Can you work these out from the model? Positions are in its coordinate system, mm. Face numbers are marked on the shaded views. Give positions to 0.01 mm unless a question says otherwise; leave off trailing zeros. Write each loop counter-clockwise with the first axis right and the second up, starting at its lowest first coordinate (ties: lowest second). Pieces come first, ordered by that corner, then holes. Notation, with made-up numbers: (87, -14) -> (122, -14) arc R14 ccw to (122, -4) -> close; hole circle Ø11 at (15.5, -39.75). An arc over 180 degrees is marked (long way). One line per item, written item: value.
from build123d import *

# Parameters (mm, degrees)
BASE_PLATE_R    = 1.6
EXTRUDE_1_DEPTH = 1.55
FILLET_1_R      = 1
SKETCH_1_R      = 3.25
SKETCH_1_R_2    = 3.5
EXTRUDE_2_DEPTH = 4.5
SKETCH_1_3_R    = 2.4
EXTRUDE_3_DEPTH = 2
SKETCH_1_4_R    = 2.5
EXTRUDE_4_DEPTH = 1.2


with BuildPart() as part:
    # Base plate → Extrude 1 (new body)
    with BuildSketch(Plane(origin=(0, 0, 0), x_dir=(1, 0, 0), z_dir=(0, 1, 0))):
        with BuildLine():
            ThreePointArc((-38.1, -33.9), (-36.869848481, -36.869848481), (-33.9, -38.1))
            Line((-33.9, -38.1), (33.9, -38.1))
            ThreePointArc((33.9, -38.1), (36.869848481, -36.869848481), (38.1, -33.9))
            Line((38.1, -33.9), (38.1, 33.9))
            ThreePointArc((38.1, 33.9), (36.869848481, 36.869848481), (33.9, 38.1))
            Line((33.9, 38.1), (-0.9, 38.1))
            Line((-0.9, 38.1), (-0.9, 27.4))
            ThreePointArc((-0.9, 27.4), (-2.9, 25.4), (-4.9, 27.4))
            Line((-4.9, 27.4), (-4.9, 38.1))
            Line((-4.9, 38.1), (-33.9, 38.1))
            ThreePointArc((-33.9, 38.1), (-36.869848481, 36.869848481), (-38.1, 33.9))
            Line((-38.1, 33.9), (-38.1, -33.9))
        make_face()
        with Locations(Location((-33.9, -33.9, 0), (0, 0, 90))):
            Circle(BASE_PLATE_R, mode=Mode.SUBTRACT)
        with Locations(Location((33.9, -33.9, 0), (0, 0, 90))):
            Circle(BASE_PLATE_R, mode=Mode.SUBTRACT)
        with Locations(Location((-33.9, 33.9, 0), (0, 0, 90))):
            Circle(BASE_PLATE_R, mode=Mode.SUBTRACT)
        with Locations(Location((33.9, 33.9, 0), (0, 0, 90))):
            Circle(BASE_PLATE_R, mode=Mode.SUBTRACT)
    extrude(amount=EXTRUDE_1_DEPTH)

    # Fillet 1
    fillet_1_edges = [part.edges().sort_by_distance(p)[0] for p in [
        (-0.9, 0.775, -38.1),
        (-4.9, 0.775, -38.1),
    ]]
    fillet(fillet_1_edges, radius=FILLET_1_R)

    # Sketch 1 → Extrude 2 (add)
    with BuildSketch(Plane.XZ):
        with Locations(Location((-22.7, -3.07, 0), (0, 0, 90))):
            Circle(SKETCH_1_R)
        with Locations(Location((-17.96, -15.36, 0), (0, 0, 90))):
            Circle(SKETCH_1_R_2)
        with Locations(Location((-5.01, -15.36, 0), (0, 0, 90))):
            Circle(SKETCH_1_R_2)
        with Locations(Location((-0.35, 10.415, 0), (0, 0, 90))):
            Circle(SKETCH_1_R)
        with Locations(Location((-22.7, 23.9, 0), (0, 0, 90))):
            Circle(SKETCH_1_R)
    extrude(amount=EXTRUDE_2_DEPTH)

    # Sketch 1_3 → Extrude 3 (add)
    with BuildSketch(Plane.XZ):
        with BuildLine():
            Line((8.9, 2), (8.9, -7.4))
            ThreePointArc((8.9, -7.4), (11.4, -9.9), (13.9, -7.4))
            Line((13.9, -7.4), (13.9, 2))
            ThreePointArc((13.9, 2), (11.4, 4.5), (8.9, 2))
        make_face()
        with BuildLine():
            Line((21.6, -0.16), (21.6, -5.24))
            ThreePointArc((21.6, -5.24), (24.1, -7.74), (26.6, -5.24))
            Line((26.6, -5.24), (26.6, -0.16))
            ThreePointArc((26.6, -0.16), (24.1, 2.34), (21.6, -0.16))
        make_face()
        with Locations(Location((16.7, -15.1, 0), (0, 0, 90))):
            Circle(SKETCH_1_3_R)
        with Locations(Location((31.9, -15.1, 0), (0, 0, 90))):
            Circle(SKETCH_1_3_R)
    extrude(amount=EXTRUDE_3_DEPTH)

    # Sketch 1_4 → Extrude 4 (add)
    with BuildSketch(Plane.XZ):
        with BuildLine():
            Line((18.761087935, -21.148507703), (17.361087935, -24.148507703))
            ThreePointArc((17.361087935, -24.148507703), (18.448507703, -27.138912065), (21.438912065, -26.051492297))
            Line((21.438912065, -26.051492297), (22.838912065, -23.051492297))
            ThreePointArc((22.838912065, -23.051492297), (21.751492297, -20.061087935), (18.761087935, -21.148507703))
        make_face()
        with BuildLine():
            ThreePointArc((22.15, -33.1), (24.4, -35.35), (26.65, -33.1))
            Line((26.65, -33.1), (26.65, -28.1))
            ThreePointArc((26.65, -28.1), (24.4, -25.85), (22.15, -28.1))
            Line((22.15, -28.1), (22.15, -33.1))
        make_face()
        with BuildLine():
            Line((21.65, -38.1), (21.65, -37.1))
            Line((21.65, -37.1), (21.65, -36.1))
            ThreePointArc((21.65, -36.1), (20.560909108, -34.172620939), (18.347964405, -34.111100529))
            ThreePointArc((18.347964405, -34.111100529), (17.472620939, -34.939090892), (17.15, -36.1))
            Line((17.15, -36.1), (17.15, -38.1))
            Line((17.15, -38.1), (21.65, -38.1))
        make_face()
        with BuildLine():
            Line((17.1, 21.71), (17.1, 14.09))
            ThreePointArc((17.1, 14.09), (19.6, 11.59), (22.1, 14.09))
            Line((22.1, 14.09), (22.1, 21.71))
            ThreePointArc((22.1, 21.71), (19.6, 24.21), (17.1, 21.71))
        make_face()
        with Locations(Location((27.7, 17.9, 0), (0, 0, 90))):
            Circle(SKETCH_1_4_R)
        with BuildLine():
            Line((38.1, -20.6), (30.8, -20.6))
            ThreePointArc((30.8, -20.6), (29.3, -22.1), (30.8, -23.6))
            Line((30.8, -23.6), (38.1, -23.6))
            Line((38.1, -23.6), (38.1, -20.6))
        make_face()
    extrude(amount=EXTRUDE_4_DEPTH)


solid = part.part
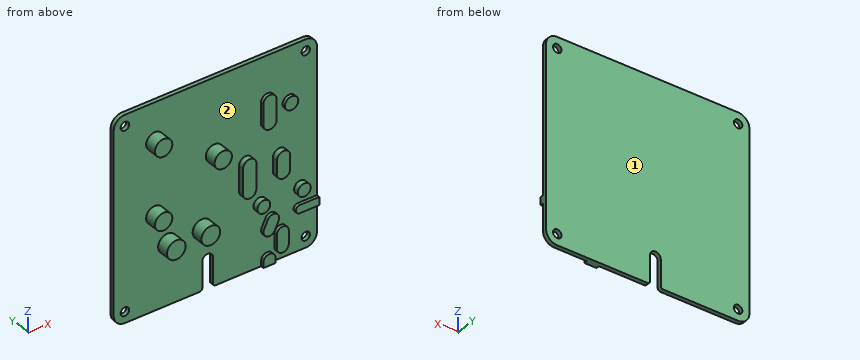
1) If we section it at A-A (y = -3): Write out the boundary of the cut face in (x, z) (3 decimals), and give its area (3 significant figures).
Answer list:
outline: circle Ø6.5 at (-22.7, -3.07); circle Ø6.5 at (-22.7, 23.9); circle Ø7 at (-17.96, -15.36); circle Ø7 at (-5.01, -15.36); circle Ø6.5 at (-0.35, 10.415)
area: 177 mm^2
2) I need wall thicknesses on L1, parallel to Z at x = 33.9, y = 0.8; L2, parallel to X at y = 0.4, z = -33.9. Which ranges of each line are inside material? Lowest first, please.
Answer list:
L1: z = -38.1 to -35.5, -32.3 to 32.3, 35.5 to 38.1
L2: x = -38.1 to -35.5, -32.3 to -4.9, -0.9 to 32.3, 35.5 to 38.1
3) Will these pins go through, and if not, where does the flat tip stop? pin 1 (8 mm diameter, centred on x = -12, z = 16.5, fed in from -Y); pin 2 (5 mm diameter, centred on x = 33.9, z = 33.9, fed in from +Y); pin 3 (2.5 mm diameter, centred on x = 11, z = -6.5, fed in from -Y); pin 4 (4 mm diameter, centred on x = 17, z = -20.5, fed in from -Y).
Answer list:
pin 1: stops at y = 0
pin 2: stops at y = 1.55
pin 3: stops at y = -2
pin 4: stops at y = -1.2
4) If we section it at B-B (x = 27.7): Write out the boundary of the cut face in (y, z), and give its area (3 significant figures).
Answer list:
outline: (-1.2, 15.4) -> (0, 15.4) -> (0, -38.1) -> (1.55, -38.1) -> (1.55, 38.1) -> (0, 38.1) -> (0, 20.4) -> (-1.2, 20.4) -> close
area: 124 mm^2
5) We'd pull the mould along X, two halves only. Please class the marked faces 1 and 2: released by +X, released by -X, zero draft, split by the parting line, or undercut.
Answer list:
face 1: zero draft
face 2: undercut
6) If we section it at D-D (x = -22.7): Write out the boundary of the cut face in (y, z).
Answer list:
outline: (-4.5, -6.32) -> (0, -6.32) -> (0, -38.1) -> (1.55, -38.1) -> (1.55, 38.1) -> (0, 38.1) -> (0, 27.15) -> (-4.5, 27.15) -> (-4.5, 20.65) -> (0, 20.65) -> (0, 0.18) -> (-4.5, 0.18) -> close
7) If we section it at C-C (z = -3.07): Write out the boundary of the cut face in (x, y).
Answer list:
outline: (-38.1, 0) -> (-25.95, 0) -> (-25.95, -4.5) -> (-19.45, -4.5) -> (-19.45, 0) -> (8.9, 0) -> (8.9, -2) -> (13.9, -2) -> (13.9, 0) -> (21.6, 0) -> (21.6, -2) -> (26.6, -2) -> (26.6, 0) -> (38.1, 0) -> (38.1, 1.55) -> (-38.1, 1.55) -> close
